Source: CAD feature listing. Evaluate the final solid. Frame: model axes, mm. Face numbers are marked on the shaded views. A direction names the side the tool comes from. Give positions to 0.01 mm unless a question says otherwise; leave off trailing zeros. Loops run counter-clockwise (first coordinate to the right, second up) from the corner with the lowest first, then second, coordinate; pieces in that order, holes last. Notation, with made-up numbers: M -8,-4.75 L 49,-4.75 A15 cw 49,9.25 Z; hole C -31,41.5 d6. An arc over 180 degrees is marked long. Answer in a Markdown table with one row per item.
```python
from build123d import *

# Parameters (mm, degrees)
SKETCH_1_R          = 10
EXTRUDE_1_DEPTH     = 27
SKETCH_3_W          = 10
SKETCH_3_H          = 20
CUT_EXTRUDE_2_DEPTH = 26
SKETCH_5_R          = 10
EXTRUDE_2_DEPTH     = 34
SKETCH_4_R          = 2
CUT_EXTRUDE_3_DEPTH = 63.617888818
M3X0_5_1_REACH      = 64.618
M3X0_5_1_BORE_R     = 1.25


with BuildPart() as part:
    # ｽｹｯﾁ1 → ﾎﾞｽ - 押し出し1 (new body)
    with BuildSketch(Plane.XY):
        Circle(SKETCH_1_R)
    extrude(amount=EXTRUDE_1_DEPTH)

    # ｽｹｯﾁ3 → ｶｯﾄ - 押し出し2 (cut)
    with BuildSketch(Plane(origin=(0, 0, 0), x_dir=(-1, 0, 0), z_dir=(0, 0, -1))):
        with Locations((-5, 0)):
            Rectangle(SKETCH_3_W, SKETCH_3_H)
    extrude(amount=-CUT_EXTRUDE_2_DEPTH, mode=Mode.SUBTRACT)

    # ｽｹｯﾁ5 → ﾎﾞｽ - 押し出し2 (add)
    with BuildSketch(Plane.XY.offset(27)):
        with Locations(Location((0, 0, 0), (0, 0, 270))):
            Circle(SKETCH_5_R)
    extrude(amount=EXTRUDE_2_DEPTH)

    # ｽｹｯﾁ4 → ｶｯﾄ - 押し出し3 (cut, through all)
    with BuildSketch(Plane(origin=(0, 0, 0), x_dir=(0, 0, -1), z_dir=(1, 0, 0))):
        with Locations((-7, 0)):
            Circle(SKETCH_4_R)
    extrude(amount=-CUT_EXTRUDE_3_DEPTH, mode=Mode.SUBTRACT)

    # M3x0.5 ねじ穴1 bore → M3x0.5 ねじ穴1 (cut, up to next)
    with BuildSketch(Plane(origin=(0, 0, 0), x_dir=(-1, 0, 0), z_dir=(0, 0, -1)), mode=Mode.PRIVATE) as m3x0_5_1_sk1:
        with Locations((5, 0)):
            Circle(M3X0_5_1_BORE_R)
    m3x0_5_1_tool1 = extrude(m3x0_5_1_sk1.sketch, amount=-M3X0_5_1_REACH, mode=Mode.PRIVATE) & part.part
    add(m3x0_5_1_tool1.solids().sort_by_distance((-5, 0, 0))[0], mode=Mode.SUBTRACT)


solid = part.part
```
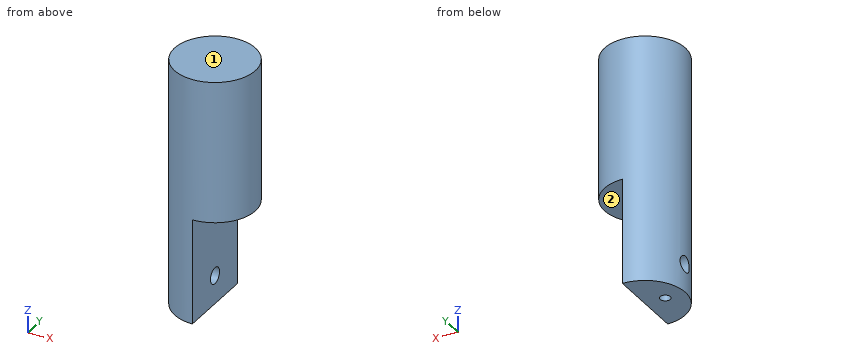
1) Set-up query: the marked faces 1 and 2. Return all of +Z, -Z, +X, -X, +Y, -Y with unobstructed straight access to the full face (end or side cutting, diameter ignored); none if empty.
Reply:
| item | result |
|---|---|
| face 1 | +Z, +X, -X, +Y, -Y |
| face 2 | -Z, +X, +Y, -Y |
2) Material intervals for L1, parallel to Z at x = -2.75, y = 0; L2, parallel to X at y = -0.5, z = 12; L3, parallel to Z at x = 4.5, y = 0, sorted ascending.
Reply:
| item | result |
|---|---|
| L1 | z = 0 to 5, 9 to 61 |
| L2 | x = -9.99 to 0 |
| L3 | z = 26 to 61 |
3) Section C-C, the plane x = -1.25. Return loops of the section in (y, z).
Reply:
| item | result |
|---|---|
| outline | M -9.92,0 L 9.92,0 L 9.92,61 L -9.92,61 Z; hole C 0,7 d4 |
4) Pin query (flat end, axial travel): pin 1 Ø6 at (x, y) = (4, -2.5) entering from -Z; pin 2 Ø4 at (x, z) = (7, 43) entering from +Y; pin 3 Ø1.5 at (y, z) = (0.5, 17.5) entering from +X. Return the tip coordinate at first contact, or that it passes through.
Reply:
| item | result |
|---|---|
| pin 1 | stops at z = 26 |
| pin 2 | stops at y = 8.66 |
| pin 3 | stops at x = 0 |
5) Section A-A, the plane y = 0. Return loops of the section in (x, z).
Reply:
| item | result |
|---|---|
| outline | M -10,0 L -6.25,0 L -6.25,5 L -10,5 Z; M -10,9 L 0,9 L 0,26 L 10,26 L 10,61 L -10,61 Z; M -3.75,0 L 0,0 L 0,5 L -3.75,5 Z |
6) Section D-D, the plane x = -5. Return loops of the section in (y, z), then the cut area to 3 significant figures.
Reply:
| item | result |
|---|---|
| outline | M -8.66,0 L -1.25,0 L -1.25,5.44 A2 cw long 1.25,5.44 L 1.25,0 L 8.66,0 L 8.66,61 L -8.66,61 Z |
| area | 1,030 mm² |
7) Section B-B, the plane z = 7. Return loops of the section in (x, y).
Reply:
| item | result |
|---|---|
| outline | M -9.8,-2 A10 ccw 0,-10 L 0,-2 Z; M -9.8,2 L 0,2 L 0,10 A10 ccw Z |
